Can you work these out from the model? Positions are in its coordinate system, mm. Face numbers are marked on the shaded views. A direction names the side the tool comes from. Give positions to 0.01 mm unless a question says otherwise; leave off trailing zeros. Write each loop counter-clockwise with the first axis right and the second up, starting at its lowest first coordinate (ties: lowest second). Pieces come first, ordered by that corner, then holes.
1. Suppose I cut it at C-C (y = 34.5). Please give me the cut outline in (x, z).
2. If I drill on probe 1 along X at (y, z) = (54.75, 3.15); probe 2 along Z at (x, y) = (-35, 9); probe 3 along X at (y, z) = (-20, -1), over which ranges is the centre line in solid material (lowest first)?
3. I'm going to push flat-ended pins straight in: pin 1 (5 mm diameter, centred on x = 17, z = -7.5, fed in from +Y); pin 2 (7.5 mm diameter, centred on y = -28.5, z = -1.5, fed in from +X); pin 3 (17.5 mm diameter, centred on x = -57, y = 35, fed in from -Z). Where does each tip first touch, or does it pass through?
4. Suppose I cut it at A-A (y = -9). Please give me the cut outline in (x, z).
5. Suppose I cut it at B-B (z = -1.7). Please give me the cut outline in (x, y), and give its area (3 significant figures).
6. Suppose I cut it at D-D (z = -8.25). Please give me the cut outline in (x, y).
7. On a 3-axis mill with a long thin cutter (end or side, diameter ignored), from which of +Z, -Z, +X, -X, +Y, -Y can I reach the whole of each face in a straight line? I mean the marked faces 1, 2, 3, 4 and 5. Say none if no direction works.
```python
from build123d import *

# Parameters (mm, degrees)
SKETCH1_W           = 93
SKETCH1_H           = 100
BOSS_EXTRUDE2_DEPTH = 6.3
SKETCH3_W           = 40
SKETCH3_H           = 100
BOSS_EXTRUDE3_DEPTH = 9.9
SKETCH4_W           = 16.2
SKETCH4_H           = 15
BOSS_EXTRUDE4_DEPTH = 24
SKETCH5_R           = 2
CUT_EXTRUDE1_DEPTH  = 50
SKETCH6_R           = 7.5
CUT_EXTRUDE2_DEPTH  = 50
SKETCH7_R           = 8
CUT_EXTRUDE3_DEPTH  = 50
EXTRUDE_THIN1_START = -5.3
SKETCH7_2_R         = 8
SKETCH7_2_R_2       = 6
EXTRUDE_THIN1_DEPTH = 1
EXTRUDE_THIN2_START = -15.2
SKETCH6_2_R         = 7.5
SKETCH6_2_R_2       = 5.5
EXTRUDE_THIN2_DEPTH = 1
SKETCH8_R           = 1.4
CUT_EXTRUDE4_DEPTH  = 20
SKETCH9_W           = 40
SKETCH9_H           = 70
CUT_EXTRUDE5_DEPTH  = 9.9
SKETCH10_R          = 1.4
CUT_EXTRUDE6_DEPTH  = 15


with BuildPart() as part:
    # Sketch1 → Boss-Extrude2 (new body)
    with BuildSketch(Plane.XY):
        with Locations((-29.68705036, 14.928057554)):
            Rectangle(SKETCH1_W, SKETCH1_H)
    extrude(amount=BOSS_EXTRUDE2_DEPTH)

    # Sketch3 → Boss-Extrude3 (add)
    with BuildSketch(Plane(origin=(0, 0, 0), x_dir=(-1, 0, 0), z_dir=(0, 0, -1))):
        with Locations((3.18705036, 14.928057554)):
            Rectangle(SKETCH3_W, SKETCH3_H)
    extrude(amount=BOSS_EXTRUDE3_DEPTH)

    # Sketch4 → Boss-Extrude4 (add)
    with BuildSketch(Plane(origin=(16.81294964, 0, 0), x_dir=(0, 0, -1), z_dir=(1, 0, 0))):
        with Locations((1.8, -12.571942446)):
            Rectangle(SKETCH4_W, SKETCH4_H)
    extrude(amount=BOSS_EXTRUDE4_DEPTH)

    # Sketch5 → Cut-Extrude1 (cut)
    with BuildSketch(Plane(origin=(0, -5.071942446, 0), x_dir=(1, 0, 0), z_dir=(0, 1, 0))):
        with Locations(Location((26.81294964, 1.7, 0), (0, 0, 180))):
            Circle(SKETCH5_R)
    extrude(amount=-CUT_EXTRUDE1_DEPTH, mode=Mode.SUBTRACT)

    # Sketch6 → Cut-Extrude2 (cut)
    with BuildSketch(Plane(origin=(0, 0, -9.9), x_dir=(-1, 0, 0), z_dir=(0, 0, -1))):
        with Locations((-1.81294964, -24.571942446)):
            Circle(SKETCH6_R)
    extrude(amount=-CUT_EXTRUDE2_DEPTH, mode=Mode.SUBTRACT)

    # Sketch7 → Cut-Extrude3 (cut)
    with BuildSketch(Plane(origin=(0, 0, 0), x_dir=(-1, 0, 0), z_dir=(0, 0, -1))):
        with Locations((53.18705036, 36.928057554)):
            Circle(SKETCH7_R)
    extrude(amount=-CUT_EXTRUDE3_DEPTH, mode=Mode.SUBTRACT)

    # Sketch7<2> → Extrude-Thin1 (add)
    with BuildSketch(Plane(origin=(0, 0, 0), x_dir=(-1, 0, 0), z_dir=(0, 0, -1)).offset(EXTRUDE_THIN1_START)):
        with Locations((53.18705036, 36.928057554)):
            Circle(SKETCH7_2_R)
        with Locations((53.18705036, 36.928057554)):
            Circle(SKETCH7_2_R_2, mode=Mode.SUBTRACT)
    extrude(amount=-EXTRUDE_THIN1_DEPTH)

    # Sketch6<2> → Extrude-Thin2 (add)
    with BuildSketch(Plane(origin=(0, 0, -9.9), x_dir=(-1, 0, 0), z_dir=(0, 0, -1)).offset(EXTRUDE_THIN2_START)):
        with Locations((-1.81294964, -24.571942446)):
            Circle(SKETCH6_2_R)
        with Locations((-1.81294964, -24.571942446)):
            Circle(SKETCH6_2_R_2, mode=Mode.SUBTRACT)
    extrude(amount=-EXTRUDE_THIN2_DEPTH)

    # Sketch8 → Cut-Extrude4 (cut)
    with BuildSketch(Plane(origin=(0, 64.928057554, 0), x_dir=(1, 0, 0), z_dir=(0, 1, 0))):
        with Locations(Location((-15.68705036, 1.8, 0), (0, 0, 270))):
            Circle(SKETCH8_R)
        with Locations(Location((9.31294964, 1.8, 0), (0, 0, 270))):
            Circle(SKETCH8_R)
    extrude(amount=-CUT_EXTRUDE4_DEPTH, mode=Mode.SUBTRACT)

    # Sketch9 → Cut-Extrude5 (cut)
    with BuildSketch(Plane(origin=(0, 0, -9.9), x_dir=(-1, 0, 0), z_dir=(0, 0, -1))):
        with Locations((3.18705036, 29.928057554)):
            Rectangle(SKETCH9_W, SKETCH9_H)
    extrude(amount=-CUT_EXTRUDE5_DEPTH, mode=Mode.SUBTRACT)

    # Sketch10 → Cut-Extrude6 (cut)
    with BuildSketch(Plane(origin=(0, 64.928057554, 0), x_dir=(1, 0, 0), z_dir=(0, 1, 0))):
        with Locations(Location((11.81294964, -3.15, 0), (0, 0, 270))):
            Circle(SKETCH10_R)
        with Locations(Location((-13.18705036, -3.15, 0), (0, 0, 270))):
            Circle(SKETCH10_R)
    extrude(amount=-CUT_EXTRUDE6_DEPTH, mode=Mode.SUBTRACT)


solid = part.part
```
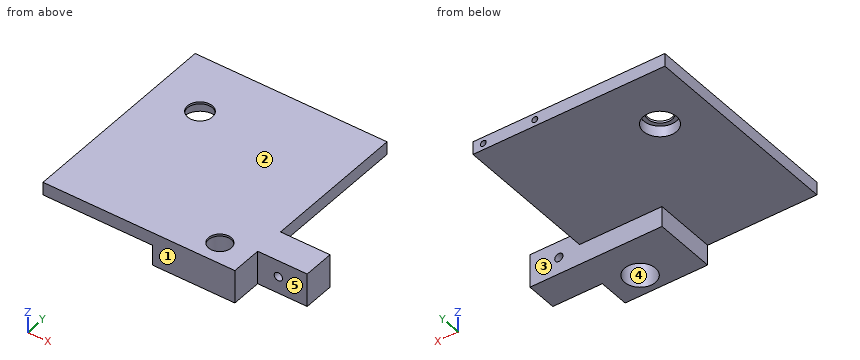
Checks:
1. outline: (-76.19, 0) - (-60.81, 0) - (-60.81, 5.3) - (-58.67, 5.3) - (-58.67, 6.3) - (-76.19, 6.3) - close; (-47.7, 5.3) - (-45.56, 5.3) - (-45.56, 0) - (16.81, 0) - (16.81, 6.3) - (-47.7, 6.3) - close
2. probe 1: x = -76.19 to -14.59, -11.79 to 10.41, 13.21 to 16.81
2. probe 2: z = 0 to 6.3
2. probe 3: x = -23.19 to -4.13, 7.76 to 24.94, 28.69 to 40.81
3. pin 1: stops at y = -5.07
3. pin 2: stops at x = 16.81
3. pin 3: stops at z = 0
4. outline: (-76.19, 0) - (-23.19, 0) - (-23.19, -9.9) - (40.81, -9.9) - (40.81, 6.3) - (-76.19, 6.3) - close; hole circle Ø4 at (26.81, -1.7)
5. outline: (-23.19, -35.07) - (16.81, -35.07) - (16.81, -20.07) - (24.81, -20.07) - (24.81, -5.07) - (-23.19, -5.07) - close; (28.81, -20.07) - (40.81, -20.07) - (40.81, -5.07) - (28.81, -5.07) - close; hole circle Ø15 at (1.81, -24.57)
5. area: 1,320 mm2
6. outline: (-23.19, -35.07) - (16.81, -35.07) - (16.81, -20.07) - (40.81, -20.07) - (40.81, -5.07) - (-23.19, -5.07) - close; hole circle Ø15 at (1.81, -24.57)
7. face 1: +Z, -Z, +X, -X, -Y
7. face 2: +Z, +X, -X, +Y, -Y
7. face 3: -Z, +X, +Y
7. face 4: -Z
7. face 5: +Z, -Z, +X, -Y
